```python
from build123d import *

# Parameters (mm, degrees)
BOSS_EXTRUDE1_DEPTH = 100


with BuildPart() as part:
    # Sketch1 → Boss-Extrude1 (new body)
    with BuildSketch(Plane(origin=(0, 0, 0), x_dir=(1, 0, 0), z_dir=(0, 1, 0))):
        Polygon((-87, 3.7), (-53.6, 3.7), (-53.6, 2.2), (-42.75, 2.2), (-42.75, 3.7), (-14.25, 3.7), (-14.25, 1.58), (-5.25, 1.58), (-5.25, 3.7), (-5.25, 6.35), (0, 6.35), (0, 0), (-18.37, 0), (-18.37, 2.44), (-27.53, 2.44), (-27.53, 0), (-63.7, 0), (-63.7, 1.2), (-72.62, 1.2), (-72.62, 0), (-79, 0), (-79, 2), (-87, 2), align=None)
    extrude(amount=BOSS_EXTRUDE1_DEPTH)


solid = part.part
```
Geometry: final body of the model. Coordinates: model frame, mm. A direction names the side the tool comes from. Round coordinates to 2 decimals unless told otherwise and drop trailing zeros. Order: outer loops, then holes, each group sorted by start corner. A loop starts at its lowest first (then second) coordinate and runs counter-clockwise, first axis right, second up. Notation, with made-up numbers: (-27.5, -14) - (28.5, -14) arc R19 ccw to (28.5, 8) - close; hole circle Ø2 at (28, 23). An arc over 180 degrees is marked (long way). Write item = value, one per line. Start each with the question number.
Q1. Pull-direction query (X, two-part tool) for faces 1 (the flat face through (-79, 49, -1)), 2 (the flat face through (-27.53, 49, -1)), 3 (the flat face through (-68, 49, -1.2)), 4 (the flat face through (-3, 49, -6.35)); classes: +X half, -X half, draft (parallel to the pull), parting line (faces both ways), or undercut.
Q2. Access query for faces 5 (the flat face through (-83, 49, -2)), 6 (the flat face through (-71, 49, -3.7)), 7 (the flat face through (-23, 49, -2.44)), 8 (the flat face through (-14.25, 49, -3)). Directions: +Z, -Z, +X, -X, +Y, -Y. A direction counts if a zero-diameter tool reaches every point of the face in a straight line with its end or side. Return the directions, or none.
Q3. Pin query (flat end, axial travel): pin 1 (5.5 mm diameter, centred on x = -46, y = 65, fed in from -Z); pin 2 (2.5 mm diameter, centred on x = -23.5, y = 74, fed in from +Z); pin 3 (1 mm diameter, centred on x = -76.5, y = 53.5, fed in from -Z). Return the tip coordinate at first contact, or that it passes through.
Q4. Ray query, line 1 (X direction, y = 40.5, z = -3); line 2 (X direction, y = 38, z = -2.25); line 3 (X direction, y = 7.5, z = -1.75). Return the intervals inside material, ascending. Write a range as from..to.
Q5. Cut plane A-A on y = 38.5. Return the cut outline in (x, z), and give its area (3 significant figures).
Q6. Cut plane B-B on z = -5.25. Return the cut outline in (x, y).
Q7. Cut plane C-C on x = -81. Return the cut outline in (y, z), and give its area (3 significant figures).
Outcome:
q1.face_1 = -X half
q1.face_2 = undercut
q1.face_3 = undercut
q1.face_4 = draft
q2.face_5 = +Z, -X, +Y, -Y
q2.face_6 = -Z, -X, +Y, -Y
q2.face_7 = +Z, +Y, -Y
q2.face_8 = -Z, +Y, -Y
q3.pin_1 = -2.2
q3.pin_2 = -2.44
q3.pin_3 = -3.7
q4.line_1 = -87..-53.6, -42.75..-14.25, -5.25..0
q4.line_2 = -87..-53.6, -42.75..-27.53, -18.37..-14.25, -5.25..0
q4.line_3 = -79..-27.53, -18.37..-14.25, -5.25..0
q5.outline = (-87, -3.7) - (-53.6, -3.7) - (-53.6, -2.2) - (-42.75, -2.2) - (-42.75, -3.7) - (-14.25, -3.7) - (-14.25, -1.58) - (-5.25, -1.58) - (-5.25, -6.35) - (0, -6.35) - (0, 0) - (-18.37, 0) - (-18.37, -2.44) - (-27.53, -2.44) - (-27.53, 0) - (-63.7, 0) - (-63.7, -1.2) - (-72.62, -1.2) - (-72.62, 0) - (-79, 0) - (-79, -2) - (-87, -2) - close
q5.area = 251 mm^2
q6.outline = (-5.25, 0) - (0, 0) - (0, 100) - (-5.25, 100) - close
q7.outline = (0, -3.7) - (100, -3.7) - (100, -2) - (0, -2) - close
q7.area = 170 mm^2
